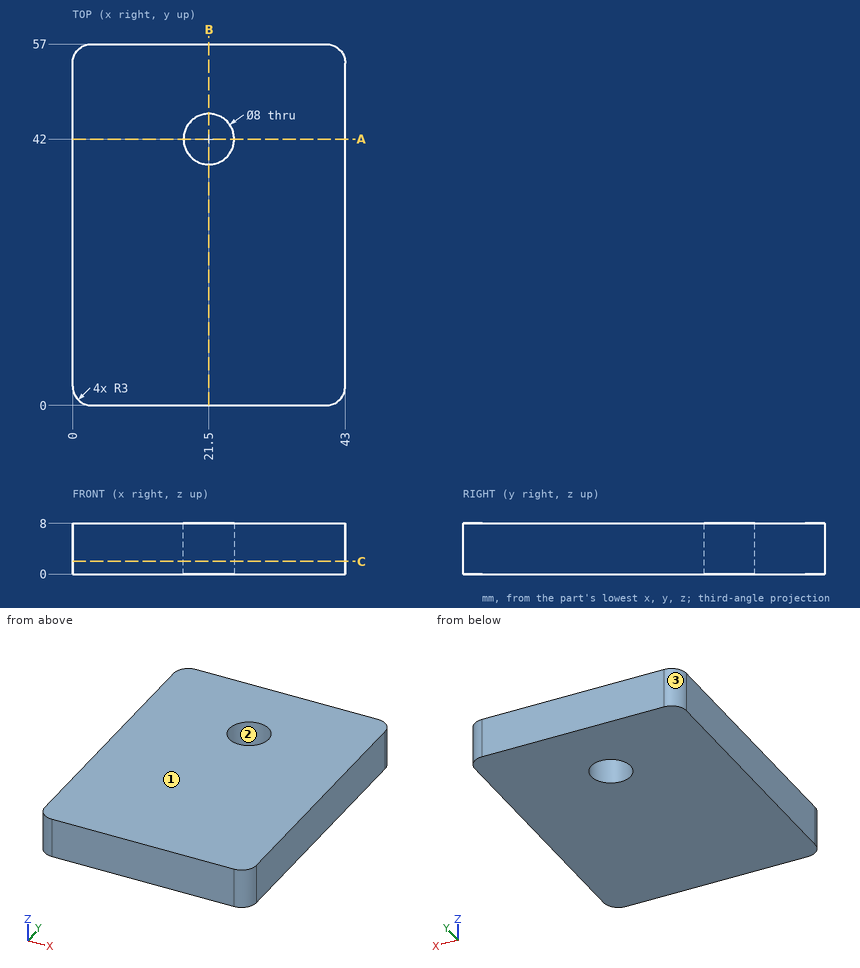
Part print with two shaded views. Sizes in mm from the minimum x, y, z corner. Coordinates: 2 decimals unless noted, no trailing zeros. Write each loop counter-clockwise with the first axis right and the second up, starting at its lowest first coordinate (ties: lowest second). Pieces come first, ordered by that corner, then holes. Notation, with made-up numbers: M 73,6 L 118,6 A29 ccw 118,38 Z; hole C -31,35 d3. An arc over 180 degrees is marked long. Return JSON: item names as keys, results as strings.
Item 1: Two-plate mould, pull along Y, no slides. Class the marked faces 1, 2 and 3: +Y half, -Y half, draft (parallel to the pull), parting line (faces both ways), or undercut.
Findings below:
{"face 1": "draft", "face 2": "undercut", "face 3": "+Y half"}
Item 2: Probe line 1 (Y direction, x = 21.5, z = 3.25); line 2 (X direction, y = 41.5, z = 0.5); line 3 (X direction, y = 54.5, z = 1.75). List the from-to ranges inside material, lowest first. Write a range as from..to.
Findings below:
{"line 1": "y = 0..38, 46..57", "line 2": "x = 0..17.53, 25.47..43", "line 3": "x = 0.04..42.96"}
Item 3: Slice it at A-A, the plane y = 42. Write the cut outline in (x, z).
Findings below:
{"outline": "M 0,0 L 17.5,0 L 17.5,8 L 0,8 Z; M 25.5,0 L 43,0 L 43,8 L 25.5,8 Z"}
Item 4: Slice it at B-B, the plane x = 21.5. Write the cut outline in (y, z), and give its area (3 significant figures).
Findings below:
{"outline": "M 0,0 L 38,0 L 38,8 L 0,8 Z; M 46,0 L 57,0 L 57,8 L 46,8 Z", "area": "392 mm2"}
Item 5: Slice it at C-C, the plane z = 2. Write the cut outline in (x, y), and give its area (3 significant figures).
Findings below:
{"outline": "M 0,3 A3 ccw 3,0 L 40,0 A3 ccw 43,3 L 43,54 A3 ccw 40,57 L 3,57 A3 ccw 0,54 Z; hole C 21.5,42 d8", "area": "2,390 mm2"}
